```python
from build123d import *

# Parameters (mm, degrees)
BOSS_EXTRUDE1_DEPTH = 50
SKETCH2_W           = 20
SKETCH2_H           = 1.5
BOSS_EXTRUDE2_DEPTH = 100
SKETCH3_W           = 15
SKETCH3_H           = 15
BOSS_EXTRUDE3_DEPTH = 1.5


with BuildPart() as part:
    # Sketch1 → Boss-Extrude1 (new body, symmetric)
    with BuildSketch(Plane(origin=(0, 0, 0), x_dir=(0, 0, -1), z_dir=(1, 0, 0))):
        Polygon((-75, 0), (0, 16.5), (0, 0), align=None)
    extrude(amount=BOSS_EXTRUDE1_DEPTH, both=True)

    # Sketch2 → Boss-Extrude2 (add)
    with BuildSketch(Plane(origin=(50, 0, 0), x_dir=(0, 0, -1), z_dir=(1, 0, 0))):
        with Locations((10, 0.75)):
            Rectangle(SKETCH2_W, SKETCH2_H)
    extrude(amount=-BOSS_EXTRUDE2_DEPTH)

    # Sketch3 → Boss-Extrude3 (add)
    with BuildSketch(Plane.XZ):
        with Locations((57.5, 27.5)):
            Rectangle(SKETCH3_W, SKETCH3_H)
        with Locations((-57.5, 27.5)):
            Rectangle(SKETCH3_W, SKETCH3_H)
    extrude(amount=-BOSS_EXTRUDE3_DEPTH)


solid = part.part
```
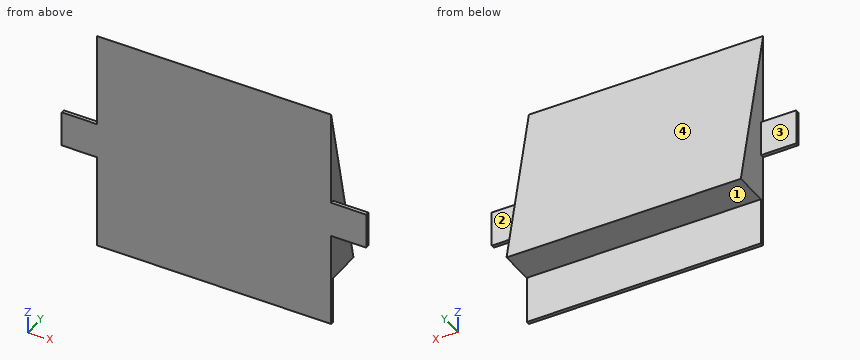
Design review of the part built by this model. Coordinates are the model's own, in mm. Face numbers are marked on the shaded views. A direction names the side the tool comes from. Coordinates: 2 decimals unless noted, no trailing zeros. Write each loop counter-clockwise with the first axis right and the second up, starting at its lowest first coordinate (ties: lowest second). Pieces come first, ordered by that corner, then holes. Notation, with made-up numbers: M 56,-14.75 L 105,-14.75 A31 ccw 105,14.25 Z; hole C 33,-22.5 d8. An arc over 180 degrees is marked long. Answer as a JSON object with one key per item and string values.
Item 1: Add section A-A, the plane z = 31. Give the boundary of the cut face in (x, y).
Outcome:
{"outline": "M -65,0 L 65,0 L 65,1.5 L 50,1.5 L 50,9.68 L -50,9.68 L -50,1.5 L -65,1.5 Z"}
Item 2: Add section B-B, the plane x = 30. Give the boundary of the cut face in (y, z).
Outcome:
{"outline": "M 0,-20 L 1.5,-20 L 1.5,0 L 16.5,0 L 0,75 Z"}
Item 3: Add section D-D, the plane z = -8. Give the boundary of the cut face in (x, y), and give its area (3 significant figures).
Outcome:
{"outline": "M -50,0 L 50,0 L 50,1.5 L -50,1.5 Z", "area": "150 mm²"}
Item 4: Insertion check: pin 1 Ø4.5 at (x, y) = (14, 9) entering from -Z; pin 2 Ø1 at (x, z) = (51, 43.5) entering from +Y; pin 3 Ø16 at (x, z) = (14.5, -13) entering from +Y; pin 4 Ø1.2 at (x, y) = (56, 0.5) entering from -Z. Each pin has a flat end and moves straight along its axis. Give the tip position at first contact, or say it passes through.
Outcome:
{"pin 1": "z = 0", "pin 2": "through", "pin 3": "y = 1.5", "pin 4": "z = 20"}
Item 5: Machinability: for the marked faces 1, 2, 3 and 4, which of the approach directions +Z, -Z, +X, -X, +Y, -Y give a long, thin tool a straight path to every point of the face, cutting with its end or side? Answer none if there is none.
Outcome:
{"face 1": "-Z, +X, -X, +Y", "face 2": "+Z, -Z, +X, +Y", "face 3": "+Z, -Z, -X, +Y", "face 4": "+Z, +X, -X, +Y"}
Item 6: Add section C-C, the plane y = 4.25. Give the boundary of the cut face in (x, z), and give its area (3 significant figures).
Outcome:
{"outline": "M -50,0 L 50,0 L 50,55.68 L -50,55.68 Z", "area": "5,570 mm²"}
Item 7: Wall thickness on probe 1 along X at (y, z) = (6, 38.5); probe 2 along Y at (x, z) = (40, -4.5); probe 3 along Y at (x, z) = (21, 15.5): over which ranges is each line inside the solid? List them lowest first.
Outcome:
{"probe 1": "-50 to 50", "probe 2": "0 to 1.5", "probe 3": "0 to 13.09"}
